Source: three-view drawing plus pictorial views. Frame: mm from the lowest corner of the part. A direction names the side the tool comes from. Give positions to 0.01 mm unless a question says otherwise; leave off trailing zeros. Loops run counter-clockwise (first coordinate to the right, second up) from the corner with the lowest first, then second, coordinate; pieces in that order, holes last. Notation, with made-up numbers: (23, 16.25) - (66, 16.25) arc R22 ccw to (66, 44.25) - close; hole circle Ø2 at (-6, 40.5). An arc over 180 degrees is marked (long way). One line per item, written item: value.
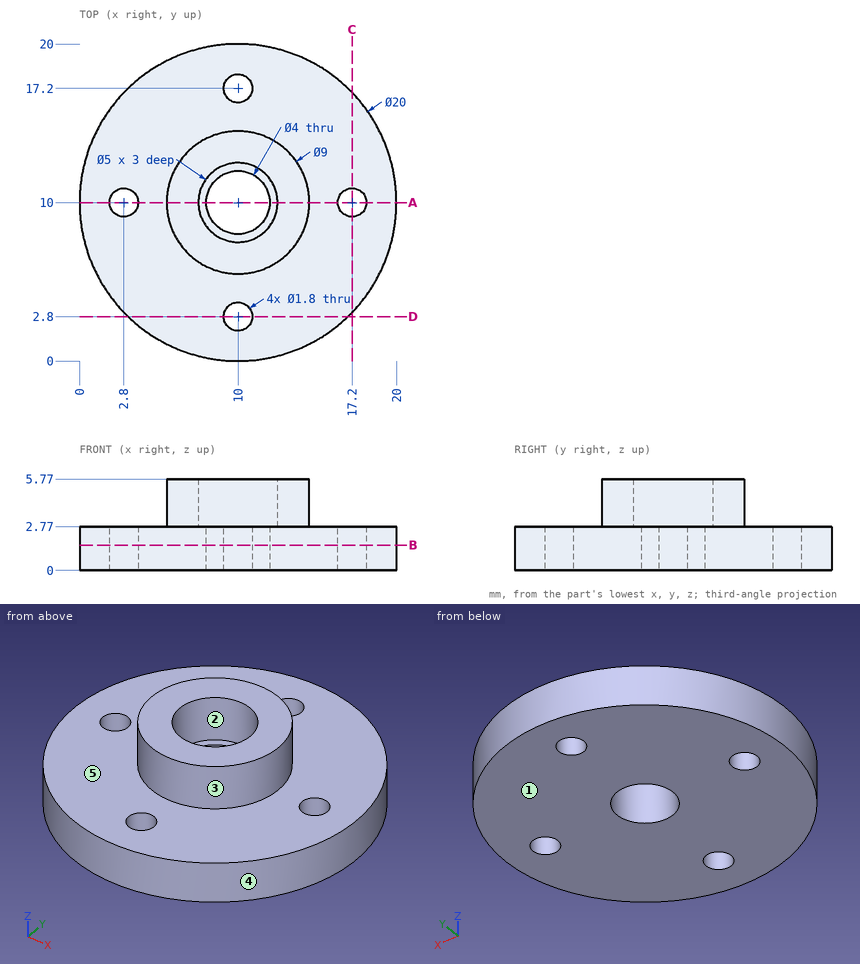
Item 1: Section C-C, the plane x = 17.2. Output: boundary loops of the cut face in (y, z), and give its area (3 significant figures).
Verdict:
outline: (3.06, 0) - (9.1, 0) - (9.1, 2.77) - (3.06, 2.77) - close; (10.9, 0) - (16.94, 0) - (16.94, 2.77) - (10.9, 2.77) - close
area: 33.5 mm^2
Item 2: Draft query along Y for the marked faces 1, 2 and 3. Return one class per face: pulls with the +Y half, pulls with the -Y half, needs draft (parallel to the pull), parting line crosses it, or undercut.
Verdict:
face 1: needs draft
face 2: undercut
face 3: parting line crosses it
Item 3: Material intervals for L1, parallel to Y at x = 10, z = 4.5; L2, parallel to Z at x = 14.5, y = 11.75; L3, parallel to Y at x = 16.75, z = 2.45, sorted ascending.
Verdict:
L1: y = 5.5 to 7.5, 12.5 to 14.5
L2: z = 0 to 2.77
L3: y = 2.62 to 9.22, 10.78 to 17.38
Item 4: Section B-B, the plane z = 1.6. Output: boundary loops of the cut face in (x, y).
Verdict:
outline: circle Ø20 at (10, 10); hole circle Ø1.8 at (2.8, 10); hole circle Ø4 at (10, 10); hole circle Ø1.8 at (10, 2.8); hole circle Ø1.8 at (10, 17.2); hole circle Ø1.8 at (17.2, 10)
Item 5: Pin query (flat end, axial travel): P1, Ø1, axis at x = 4, z = 2.5, coming from the +Y side; P2, Ø2, axis at x = 17.2, y = 10, coming from the +Z side. Return the tip coordinate at first contact, or that it passes through.
Verdict:
P1: stops at y = 18.35
P2: stops at z = 2.77
Item 6: Access query for the marked faces 4 and 5. Directions: +Z, -Z, +X, -X, +Y, -Y. A direction counts if a zero-diameter tool reaches every point of the face in a straight line with its end or side. Return the directions, or none.
Verdict:
face 4: +Z, -Z
face 5: +Z
Item 7: Section A-A, the plane y = 10. Output: boundary loops of the cut face in (x, z).
Verdict:
outline: (0, 0) - (1.9, 0) - (1.9, 2.77) - (0, 2.77) - close; (3.7, 0) - (8, 0) - (8, 2.77) - (7.5, 2.77) - (7.5, 5.77) - (5.5, 5.77) - (5.5, 2.77) - (3.7, 2.77) - close; (12, 0) - (16.3, 0) - (16.3, 2.77) - (14.5, 2.77) - (14.5, 5.77) - (12.5, 5.77) - (12.5, 2.77) - (12, 2.77) - close; (18.1, 0) - (20, 0) - (20, 2.77) - (18.1, 2.77) - close
